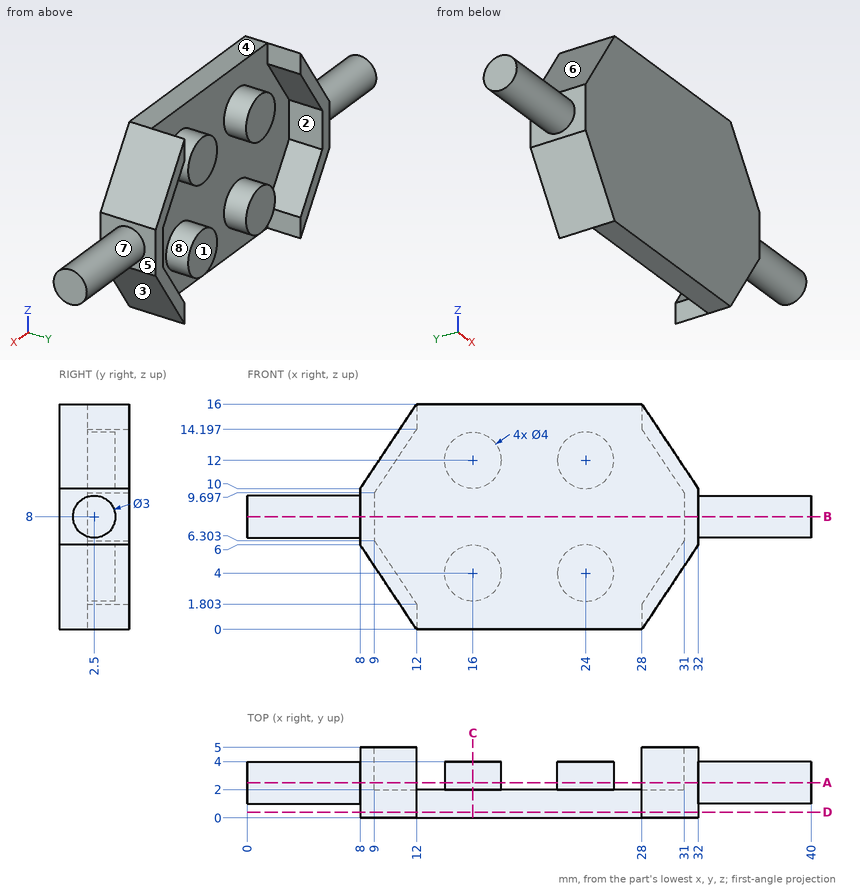
Input: dimensioned drawing with shaded views. Units: mm. Origin: part minimum x, y, z. A direction names the side the tool comes from. Coordinates: 2 decimals unless noted, no trailing zeros. Order: outer loops, then holes, each group sorted by start corner. A loop starts at its lowest first (then second) coordinate and runs counter-clockwise, first axis right, second up. Notation, with made-up numbers: (-22, 77.5) - (9, 77.5) arc R10 ccw to (9, 96.5) - close; hole circle Ø5 at (-30, 69). An arc over 180 degrees is marked (long way). Put each result on its own line as item: value.
1. Cut plane B-B on z = 8. Return the cut outline in (x, y).
Report:
outline: (0, 1) - (8, 1) - (8, 0) - (32, 0) - (32, 1) - (40, 1) - (40, 4) - (32, 4) - (32, 5) - (31, 5) - (31, 2) - (9, 2) - (9, 5) - (8, 5) - (8, 4) - (0, 4) - close
2. Cut plane C-C on x = 16. Return the cut outline in (y, z).
Report:
outline: (0, 0) - (2, 0) - (2, 2) - (4, 2) - (4, 6) - (2, 6) - (2, 10) - (4, 10) - (4, 14) - (2, 14) - (2, 16) - (0, 16) - close
3. Cut plane D-D on y = 0.4. Return the cut outline in (x, z).
Report:
outline: (8, 6) - (12, 0) - (28, 0) - (32, 6) - (32, 10) - (28, 16) - (12, 16) - (8, 10) - close
4. Line query: line 1 along X through (y, z) = (2.25, 5.75) (1 decimal); line 2 along X through (y, z) = (4.1, 7); line 3 along X through (y, z) = (3.1, 4.25) (1 decimal). Output: solid intervals per line, ascending.
Report:
line 1: x = 8.2 to 9.4, 15 to 17, 23 to 25, 30.6 to 31.8
line 2: x = 8 to 9, 31 to 32
line 3: x = 9.2 to 10.4, 14 to 18, 22 to 26, 29.6 to 30.8
5. Cut plane A-A on y = 2.5. Return the cut outline in (x, z), then the cut area to 3 significant figures.
Report:
outline: (0, 6.5) - (8, 6.5) - (8, 6) - (12, 0) - (12, 1.8) - (9, 6.3) - (9, 9.7) - (12, 14.2) - (12, 16) - (8, 10) - (8, 9.5) - (0, 9.5) - close; circle Ø4 at (16, 4); circle Ø4 at (16, 12); circle Ø4 at (24, 4); circle Ø4 at (24, 12); (28, 0) - (32, 6) - (32, 6.5) - (40, 6.5) - (40, 9.5) - (32, 9.5) - (32, 10) - (28, 16) - (28, 14.2) - (31, 9.7) - (31, 6.3) - (28, 1.8) - close
area: 131 mm2
6. Contact query for flat-ended pins moving along their axis: pin 1 Ø1.2 at (x, z) = (24, 11) entering from +Y; pin 2 Ø0.5 at (y, z) = (4, 15) entering from +X; pin 3 Ø0.5 at (y, z) = (3, 1.5) entering from +X. Output: stop coordinate, or through.
Report:
pin 1: stops at y = 4
pin 2: stops at x = 28.83
pin 3: stops at x = 29.17
7. Draft query along X for the marked faces 6, 7 and 8. Return one class per face: pulls with the +X half, pulls with the -X half, needs draft (parallel to the pull), parting line crosses it, or undercut.
Report:
face 6: pulls with the -X half
face 7: needs draft
face 8: undercut
8. Reachability of the marked faces 1, 2, 3, 4 and 5 from +Z, -Z, +X, -X, +Y, -Y: full face, straight path, thin tool, end or side. Return the list, or none.
Report:
face 1: +Z, -Z, +Y
face 2: +Y
face 3: -Z, +X, +Y, -Y
face 4: +Z, +X, -X, +Y, -Y
face 5: +X
